Autodesk Inventor part; units mm, degrees
ref_plane "YZ Plane" through (0, 0, 0) normal (1, 0, 0) x (0, 1, 0)
ref_plane "XZ Plane" through (0, 0, 0) normal (0, 1, 0) x (-1, 0, 0)
ref_plane "XY Plane" through (0, 0, 0) normal (0, 0, 1) x (1, 0, 0)
sketch "草圖1" plane through (0, 0, 0) normal (1, 0, 0) x (0, 1, 0)
  line L0 (0, 0) -> (0, -113.9)
  circle A0 centre (0, 0) radius 6
  circle A1 centre (0, -113.9) radius 6
  circle A2 centre (0, 0) radius 9
  circle A3 centre (0, -113.9) radius 9
  line L1 (5, -7.4833) -> (5, -17.4833)
  line L2 (5, -17.4833) -> (3, -19.4833)
  line L3 (3, -19.4833) -> (3, -94.4167)
  line L4 (3, -94.4167) -> (5, -96.4167)
  line L5 (5, -96.4167) -> (5, -106.4167)
  line L6 (-5, -7.4833) -> (-5, -17.4833)
  line L7 (-5, -17.4833) -> (-3, -19.4833)
  line L8 (-3, -19.4833) -> (-3, -94.4167)
  line L9 (-3, -94.4167) -> (-5, -96.4167)
  line L10 (-5, -96.4167) -> (-5, -106.4167)
  dimension "d0" = 113.9
  dimension "d1" = 12
  dimension "d2" = 12
  dimension "d3" = 18
  dimension "d4" = 18
  dimension "d5" = 3
  dimension "d6" = 3
  dimension "d7" = 135
  dimension "d8" = 5
  dimension "d9" = 10
  dimension "d10" = 10
  dimension "d11" = 135
extrude "擠出1" add sketch "草圖1" along normal mid plane 5
fillet "圓角1" radius 2 12 edges at (0, 5, -7.4833) (0, 5, -17.4833) (0, 3, -19.4833) (0, 3, -94.4167) (0, 5, -96.4167) (0, 5, -106.4167) (0, -5, -7.4833) (0, -5, -17.4833) (0, -3, -19.4833) (0, -3, -94.4167) (0, -5, -96.4167) (0, -5, -106.4167)
equation "\"d2\" = d1"
equation "\"d4\" = d3"
equation "\"d6\" = d5"
equation "\"d10\" = d9"
equation "\"d11\" = d7"
properties part number "Link_FG"
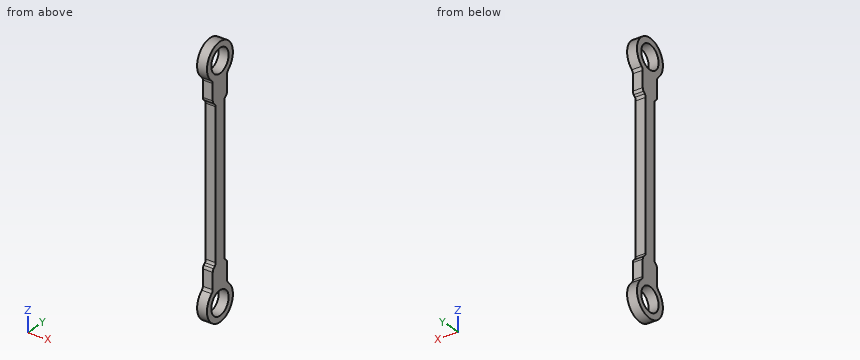
Work out the finished part from the listing and answer in its coordinate system (mm). Coordinates: 2 decimals unless noted, no trailing zeros. Order: outer loops, then holes, each group sorted by start corner. A loop starts at its lowest first (then second) coordinate and runs counter-clockwise, first axis right, second up. Notation, with made-up numbers: (57.25, -21.5) - (62.25, -21.5) arc R19 ccw to (62.25, -9.5) - close; hole circle Ø5 at (81, -6). An arc over 180 degrees is marked (long way). Put each result on its own line as item: value. Start each with the question number.
1) Find section C-C (x = 0.9). Give the vertices of the cut face in (y, z).
2) Find section D-D (z = -87). Give the vertices of the cut face in (x, y), plus the area to 3 significant figures.
3) Flat-ended cylindrical pins translate along their axes: pin 1 (2.5 mm diameter, centred on x = -1, z = -52.5, fed in from +Y); pin 2 (2.5 mm diameter, centred on x = 1, z = -54, fed in from -Y); pin 3 (1.5 mm diameter, centred on x = 0, z = -103, fed in from -Y). Find the tip coordinate at first contact, or state that the pin passes through.
4) Find the intervals of material crossed by line 1 (Z direction, x = 0, y = 0); line 2 (Y direction, x = -0.9, z = -113.9); line 3 (Z direction, x = -0.15, y = 3.75), in increasing order. Write a range as from..to.
5) Find section A-A (z = -113.9). Give the vertices of the cut face in (x, y).
6) Find section B-B (y = 0). Give the vertices of the cut face in (x, z).
Results list:
1. outline: (-5.73, -106.96) arc R9 ccw (long way) to (5.73, -106.96) arc R2 cw to (5, -105.41) - (5, -97.25) arc R2 ccw to (4.41, -95.83) - (3.59, -95) arc R2 cw to (3, -93.59) - (3, -20.31) arc R2 cw to (3.59, -18.9) - (4.41, -18.07) arc R2 ccw to (5, -16.65) - (5, -8.49) arc R2 cw to (5.73, -6.94) arc R9 ccw (long way) to (-5.73, -6.94) arc R2 cw to (-5, -8.49) - (-5, -16.65) arc R2 ccw to (-4.41, -18.07) - (-3.59, -18.9) arc R2 cw to (-3, -20.31) - (-3, -93.59) arc R2 cw to (-3.59, -95) - (-4.41, -95.83) arc R2 ccw to (-5, -97.25) - (-5, -105.41) arc R2 cw to start; hole circle Ø12 at (0, -113.9); hole circle Ø12 at (0, 0)
2. outline: (-2.5, -3) - (2.5, -3) - (2.5, 3) - (-2.5, 3) - close
2. area: 30.0 mm^2
3. pin 1: stops at y = 3
3. pin 2: stops at y = -3
3. pin 3: stops at y = -5
4. line 1: z = -122.9..-119.9, -107.9..-6, 6..9
4. line 2: y = -9..-6, 6..9
4. line 3: z = -122.08..-118.58, -109.22..-95.17, -18.73..-4.68, 4.68..8.18
5. outline: (-2.5, -9) - (2.5, -9) - (2.5, -6) - (-2.5, -6) - close; (-2.5, 6) - (2.5, 6) - (2.5, 9) - (-2.5, 9) - close
6. outline: (-2.5, -122.9) - (2.5, -122.9) - (2.5, -119.9) - (-2.5, -119.9) - close; (-2.5, -107.9) - (2.5, -107.9) - (2.5, -6) - (-2.5, -6) - close; (-2.5, 6) - (2.5, 6) - (2.5, 9) - (-2.5, 9) - close
